CAD build for the part. Positions are in the model's coordinates, mm. Face numbers are marked on the shaded views. Give positions to 0.01 mm unless a question says otherwise; leave off trailing zeros. Loops run counter-clockwise (first coordinate to the right, second up) from the corner with the lowest first, then second, coordinate; pieces in that order, holes last.
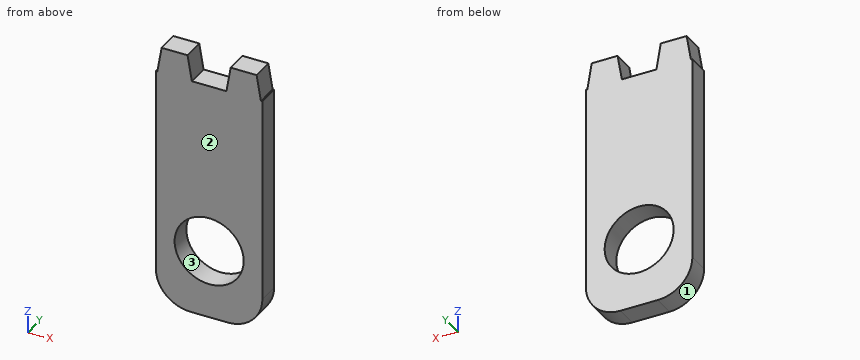
```python
from build123d import *

# Parameters (mm, degrees)
SKETCH1_W           = 30.83672877
SKETCH1_H           = 70
SKETCH1_R           = 10
BOSS_EXTRUDE1_DEPTH = 6.35
FILLET1_R           = 10


with BuildPart() as part:
    # Sketch1 → Boss-Extrude1 (new body)
    with BuildSketch(Plane(origin=(0, 0, 0), x_dir=(1, 0, 0), z_dir=(0, 1, 0))):
        Polygon((13.75, -42.5), (15, -35), (5, -35), (6.25, -42.5), align=None)
        Polygon((-5, -35), (-15, -35), (-13.75, -42.5), (-6.25, -42.5), align=None)
        Rectangle(SKETCH1_W, SKETCH1_H)
        with Locations((0, 15)):
            Circle(SKETCH1_R, mode=Mode.SUBTRACT)
    extrude(amount=BOSS_EXTRUDE1_DEPTH)

    # Fillet1
    fillet1_edges = [part.edges().sort_by_distance(p)[0] for p in [
        (-15.418364385, 3.175, -35),
        (15.418364385, 3.175, -35),
    ]]
    fillet(fillet1_edges, radius=FILLET1_R)


solid = part.part
```
1. Drop flat-ended pins along their axis: pin 1 (1.5 mm diameter, centred on x = 7, z = -13, fed in from -Y); pin 2 (1.9 mm diameter, centred on x = -1.5, y = 4.5, fed in from +Z). Give the stop position or say it passes through.
Responses:
pin 1: passes through
pin 2: stops at z = 35
2. Pull direction Z, two halves, no side cores. Call the marked faces 1, 2 and 3: released by +Z, released by -Z, zero draft, split by the parting line, or undercut.
Responses:
face 1: released by -Z
face 2: zero draft
face 3: undercut
3. Saw through at D-D, the plane x = 13. List the corners of the cut face in (y, z), and give its area (3 significant figures).
Responses:
outline: (0, -31.52) - (6.35, -31.52) - (6.35, 42.5) - (0, 42.5) - close
area: 470 mm2
4. Probe line 1 along X through (y, z) = (3, -15); line 2 along Z through (x, y) = (0, 2.25); line 3 along Z through (x, y) = (2.5, 1.75). List the from-to ranges inside material, lowest first.
Responses:
line 1: x = -15.42 to -10, 10 to 15.42
line 2: z = -35 to -25, -5 to 35
line 3: z = -35 to -24.68, -5.32 to 35
5. Saw through at A-A, the plane x = 0. List the corners of the cut face in (y, z), and give its area (4 significant figures).
Responses:
outline: (0, -35) - (6.35, -35) - (6.35, -25) - (0, -25) - close; (0, -5) - (6.35, -5) - (6.35, 35) - (0, 35) - close
area: 317.5 mm2
6. Saw through at B-B, the plane z = -15. List the corners of the cut face in (x, y), and give its area (3 significant figures).
Responses:
outline: (-15.42, 0) - (-10, 0) - (-10, 6.35) - (-15.42, 6.35) - close; (10, 0) - (15.42, 0) - (15.42, 6.35) - (10, 6.35) - close
area: 68.8 mm2
7. Saw through at C-C, the plane y = 5.5. List the corners of the cut face in (x, z).
Responses:
outline: (-15.42, -25) arc R10 ccw to (-5.42, -35) - (5.42, -35) arc R10 ccw to (15.42, -25) - (15.42, 35) - (15, 35) - (13.75, 42.5) - (6.25, 42.5) - (5, 35) - (-5, 35) - (-6.25, 42.5) - (-13.75, 42.5) - (-15, 35) - (-15.42, 35) - close; hole circle Ø20 at (0, -15)
